Answer from the drawing. Dimensions are ordinates in mm from the lowest x, y and z of the part. A direction names the side the tool comes from. Give positions to 0.01 mm unless a question says otherwise; leave off trailing zeros. Loops run counter-clockwise (first coordinate to the right, second up) from the corner with the lowest first, then second, coordinate; pieces in that order, holes last. Notation, with made-up numbers: (-26.5, 76) - (9.5, 76) arc R7 cw to (9.5, 88) - close; hole circle Ø7 at (70, -20.75). An arc over 180 degrees is marked (long way). Write each question's results on one line, items separated by ' | '. Start each with the question number.
Q1. The part is cut by section B-B, the plane y = 10.25. Write down the section's boundary in (x, z).
Q2. The part is cut by section D-D, the plane z = 7. Write down the section's boundary in (x, y), plus the area to 3 significant figures.
Q3. Given pin 1 (2 mm diameter, centred on y = 4.5, z = 33, fed in from -X); pin 2 (3 mm diameter, centred on y = 6, z = 13.5, fed in from +X); pin 3 (5.5 mm diameter, centred on y = 4.5, z = 46.5, fed in from -X), each flat-ended and moving along its own axis, determine where each tip first touches the part or whether it passes through.
Q4. Find the intervals of material crossed by line 1 (X direction, y = 5.75, z = 5); line 2 (Z direction, x = 79, y = 6); line 3 (Y direction, x = 107.95, z = 1.25), in increasing order. Write a range as from..to.
Q5. For the marked faces 1, 2, 3 and 4, determine the directions among +Z, -Z, +X, -X, +Y, -Y from which every point of the face is accessible in a straight line to the end or side of a thin tool.
Q6. The part is cut by section A-A, the plane x = 87.5. Write down the section's boundary in (y, z), plus the area to 3 significant figures.
Q7. The part is cut by section C-C, the plane x = 6.35. Write down the section's boundary in (y, z), plus the area to 3 significant figures.
Q8. Determine the mould class of the marked faces 5, 6 and 7 for opening direction Z: +Z half, -Z half, draft (parallel to the pull), parting line (faces both ways), or undercut.
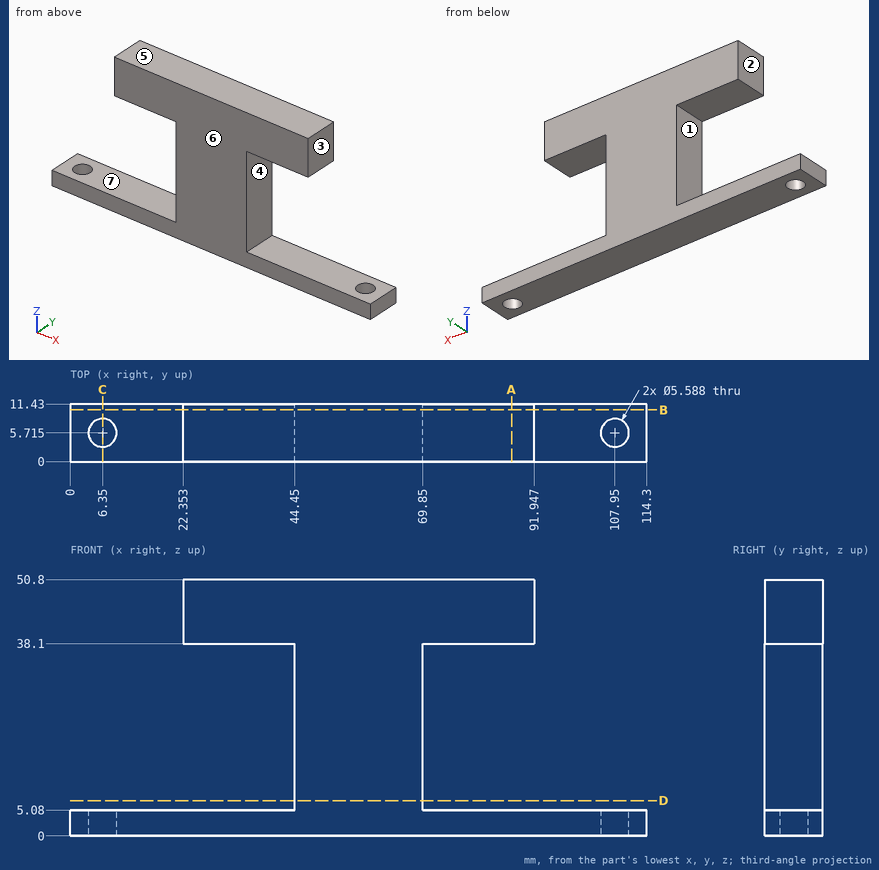
Check sheet entries:
1) outline: (0, 0) - (114.3, 0) - (114.3, 5.08) - (69.85, 5.08) - (69.85, 38.1) - (91.95, 38.1) - (91.95, 50.8) - (22.35, 50.8) - (22.35, 38.1) - (44.45, 38.1) - (44.45, 5.08) - (0, 5.08) - close
2) outline: (44.45, 0) - (69.85, 0) - (69.85, 11.43) - (44.45, 11.43) - close | area: 290 mm^2
3) pin 1: stops at x = 44.45 | pin 2: stops at x = 69.85 | pin 3: stops at x = 22.35
4) line 1: x = 0..3.56, 9.14..105.16, 110.74..114.3 | line 2: z = 0..5.08, 38.1..50.8 | line 3: y = 0..2.92, 8.51..11.43
5) face 1: -X, +Y, -Y | face 2: +Z, -X, +Y, -Y | face 3: +Z, +X, +Y, -Y | face 4: +X, +Y, -Y
6) outline: (0, 0) - (11.43, 0) - (11.43, 5.08) - (0, 5.08) - close; (0, 38.1) - (11.43, 38.1) - (11.43, 50.8) - (0, 50.8) - close | area: 203 mm^2
7) outline: (0, 0) - (2.92, 0) - (2.92, 5.08) - (0, 5.08) - close; (8.51, 0) - (11.43, 0) - (11.43, 5.08) - (8.51, 5.08) - close | area: 29.7 mm^2
8) face 5: +Z half | face 6: draft | face 7: undercut
